```python
from build123d import *

# Parameters (mm, degrees)
SKETCH1_W            = 113
SKETCH1_H            = 80
BOSS_EXTRUDE1_DEPTH  = 1.6
M3_CLEARANCE_HOLE1_D = 3.6
MIRROR2_COPY_1_D     = 3.6


with BuildPart() as part:
    # Sketch1 → Boss-Extrude1 (new body)
    with BuildSketch(Plane(origin=(0, 0, 0), x_dir=(1, 0, 0), z_dir=(0, 1, 0))):
        Rectangle(SKETCH1_W, SKETCH1_H)
    extrude(amount=BOSS_EXTRUDE1_DEPTH)

    # M3 Clearance Hole1 (through all)
    with Locations(Plane(origin=(0, 1.6, 0), x_dir=(1, 0, 0), z_dir=(0, 1, 0))):
        with Locations((-52.5, 36)):
            m3_clearance_hole1 = Hole(M3_CLEARANCE_HOLE1_D / 2)

    # Mirror1: M3 Clearance Hole1 across plane
    add(m3_clearance_hole1.mirror(Plane(origin=(0, 0, 0), x_dir=(0, 0, 1), z_dir=(1, 0, 0))), mode=Mode.SUBTRACT)

    # Mirror2: M3 Clearance Hole1 across plane
    add(m3_clearance_hole1.mirror(Plane.XY), mode=Mode.SUBTRACT)

    # Mirror2 copy 1 (through all)
    with Locations(Plane(origin=(0, 1.6, 0), x_dir=(-1, 0, 0), z_dir=(0, 1, 0))):
        with Locations((-52.5, 36)):
            Hole(MIRROR2_COPY_1_D / 2)


solid = part.part
```
For this review, take the finished solid that the model builds, in its own axes (mm). Give positions to 0.01 mm unless a question says otherwise; leave off trailing zeros. Write each loop counter-clockwise with the first axis right and the second up, starting at its lowest first coordinate (ties: lowest second). Pieces come first, ordered by that corner, then holes. Notation, with made-up numbers: M 80,-25 L 133,-25 A30 cw 133,2 Z; hole C 81.5,-37 d3. An arc over 180 degrees is marked long. One line per item, written item: value.
1) Take a section at A-A, the plane z = -36. Write out the cut boundary in (x, y), then the cut area to 3 significant figures.
Results are:
outline: M -56.5,0 L -54.3,0 L -54.3,1.6 L -56.5,1.6 Z; M -50.7,0 L 50.7,0 L 50.7,1.6 L -50.7,1.6 Z; M 54.3,0 L 56.5,0 L 56.5,1.6 L 54.3,1.6 Z
area: 169 mm²
2) Take a section at B-B, the plane x = 52.5. Write out the cut boundary in (y, z), then the cut area to 3 significant figures.
Results are:
outline: M 0,-40 L 1.6,-40 L 1.6,-37.8 L 0,-37.8 Z; M 0,-34.2 L 1.6,-34.2 L 1.6,34.2 L 0,34.2 Z; M 0,37.8 L 1.6,37.8 L 1.6,40 L 0,40 Z
area: 116 mm²
3) The part is to be moulded in two halves that separate along Z. For faces 1 (the cylindrical face through (52.266, 0.789, 37.785)), 2 (the cylindrical face through (-52.266, 0.789, -37.785)), 3 (the flat face through (-1, 1.6, -1)), say which applies: +Z half, -Z half, draft (parallel to the pull), parting line (faces both ways), or undercut.
Results are:
face 1: undercut
face 2: undercut
face 3: draft
4) For line 1 (Z direction, x = -52.5, y = 1); line 2 (Z direction, x = -51.5, y = 1.15), list the stretches that pass through material, from the lowest coordinate up. Write a range as from..to.
Results are:
line 1: z = -40..-37.8, -34.2..34.2, 37.8..40
line 2: z = -40..-37.5, -34.5..34.5, 37.5..40
